Geometry check sheet. Reference: the model listing, model coordinates, mm. A direction names the side the tool comes from. Give positions to 0.01 mm unless a question says otherwise; leave off trailing zeros. Loops run counter-clockwise (first coordinate to the right, second up) from the corner with the lowest first, then second, coordinate; pieces in that order, holes last. Notation, with made-up numbers: (79, 31.5) -> (91, 31.5) arc R31 cw to (91, 57.5) -> close; hole circle Ø1 at (89.25, 56). An arc over 180 degrees is marked (long way). Write each question's results on one line, items separated by ' | '. Start each with the question number.
1) Set-up check for faces 1 (the face through (0, 9, 85)), 2 (the face through (0, -17, -82)), 3 (the face through (-5, 9, 1)), 4 (the face through (0, -17, 82)): record each of +Z, -Z, +X, -X, +Y, -Y from which the full face is reachable in a straight line by a thin tool's end or side.
2) Sectioned sample at B-B on z = -49. Record the cut outline in (x, y).
3) Scan lines: line 1 (Y direction, x = -9.5, z = 34); line 2 (Z direction, x = 0.5, y = 4); line 3 (Y direction, x = 12.25, z = 79.5). Record each from-to range of solid material in increasing order. Write a range as from..to.
4) Depth check by flat-ended pin: pin 1 (3 mm diameter, centred on x = -1, y = 15, fed in from +Z); pin 2 (9.5 mm diameter, centred on y = 9, z = 20.5, fed in from +X); pin 3 (2 mm diameter, centred on x = 2, y = 11, fed in from -Z). Enter the tip coordinate at first touch or a pass-through.
5) Sectioned sample at C-C on y = 8.5. Record the cut outline in (x, z), then the cut area to 3 significant figures.
6) Sectioned sample at A-A on x = 12.5. Record the cut outline in (y, z).
```python
from build123d import *

# Parameters (mm, degrees)
SKETCH_W        = 30
SKETCH_H        = 50
PAD_DEPTH       = 180
SKETCH001_W     = 8
SKETCH001_H     = 15
SKETCH001_W_2   = 32
SKETCH001_H_2   = 5
POCKET_DEPTH    = 408.418759
SKETCH002_W     = 10
SKETCH002_H     = 32
POCKET001_DEPTH = 558.418759


with BuildPart() as part:
    # Sketch (on DatumPlane) → Pad (new body)
    with BuildSketch(Plane.XY.offset(90)):
        Rectangle(SKETCH_W, SKETCH_H)
    extrude(amount=-PAD_DEPTH)

    # Sketch001 (on DatumPlane) → Pocket (cut, through all)
    with BuildSketch(Plane.YZ.offset(15)):
        with Locations((-21, 82.5)):
            Rectangle(SKETCH001_W, SKETCH001_H)
        with Locations((9, 87.5)):
            Rectangle(SKETCH001_W_2, SKETCH001_H_2)
    pocket = extrude(amount=-POCKET_DEPTH, mode=Mode.SUBTRACT)

    # Mirrored: Pocket across XY
    add(pocket.mirror(Plane.XY), mode=Mode.SUBTRACT)

    # Sketch002 (on DatumPlane) → Pocket001 (cut, through all)
    with BuildSketch(Plane.XY.offset(90)):
        with Locations((10, 9)):
            Rectangle(SKETCH002_W, SKETCH002_H)
    pocket001 = extrude(amount=-POCKET001_DEPTH, mode=Mode.SUBTRACT)

    # Mirrored001: Pocket001 across Sketch002 V_Axis
    add(pocket001.mirror(Plane(origin=(0, 0, 90), x_dir=(0, 0, 1), z_dir=(1, 0, 0))), mode=Mode.SUBTRACT)


solid = part.part
```
Result:
1) face 1: +Z, +X, -X, +Y | face 2: -Z, +X, -X, -Y | face 3: +Z, -Z, -X, +Y | face 4: +Z, +X, -X, -Y
2) outline: (-15, -25) -> (15, -25) -> (15, -7) -> (5, -7) -> (5, 25) -> (-5, 25) -> (-5, -7) -> (-15, -7) -> close
3) line 1: -25..-7 | line 2: -85..85 | line 3: -17..-7
4) pin 1: z = 85 | pin 2: x = 5 | pin 3: z = -85
5) outline: (-5, -85) -> (5, -85) -> (5, 85) -> (-5, 85) -> close | area: 1,700 mm^2
6) outline: (-25, -75) -> (-17, -75) -> (-17, -90) -> (-7, -90) -> (-7, 90) -> (-17, 90) -> (-17, 75) -> (-25, 75) -> close
